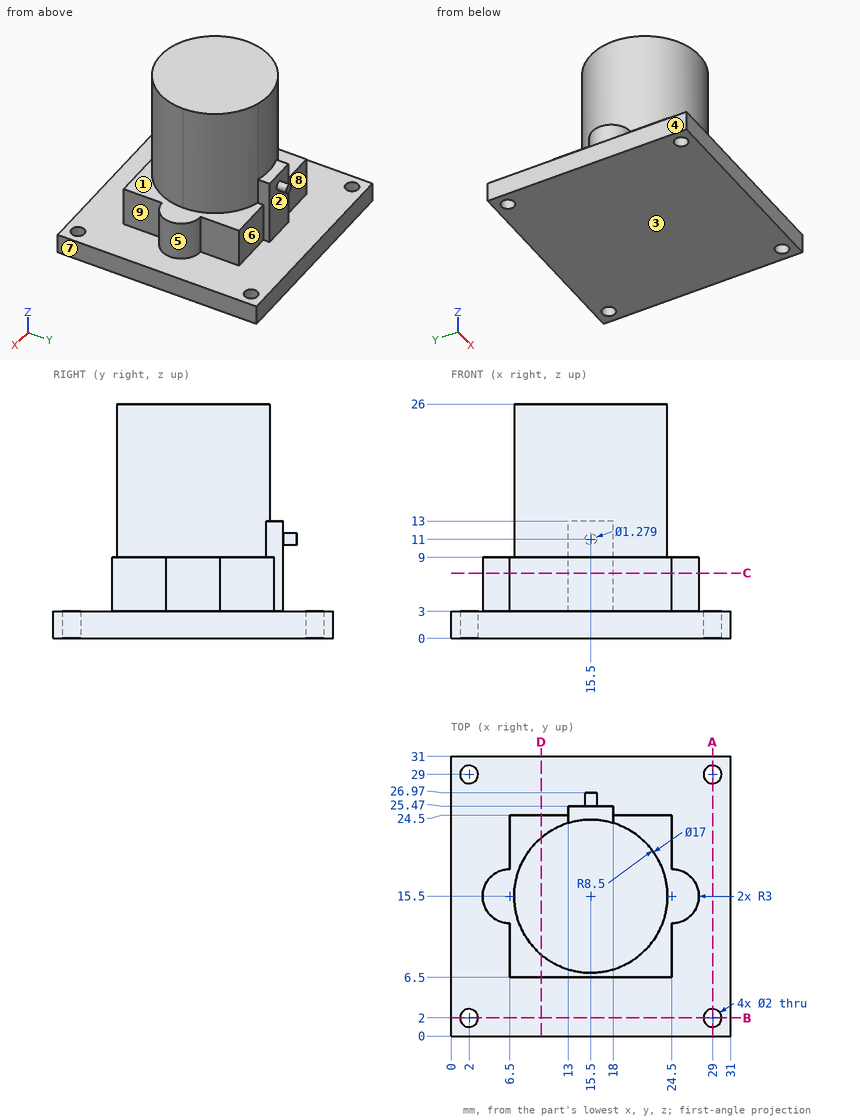
Can you work these out from the drawing? Everything is in mm from the part's minimum corner. A direction names the side the tool comes from. Coordinates: 2 decimals unless noted, no trailing zeros. Loops run counter-clockwise (first coordinate to the right, second up) from the corner with the lowest first, then second, coordinate; pieces in that order, holes last. Notation, with made-up numbers: M 20,22 L 75,22 A22 ccw 75,55 Z; hole C 31.5,5 d6. An arc over 180 degrees is marked long. Put each result on its own line as item: value. Start each with the question number.
(1) Thinking about a two-plate mould opening in Z: for the marked faces 1, 2, 3 and 4, which applies, pulls with the +Z half, pulls with the -Z half, needs draft (parallel to the pull), parting line crosses it, or undercut?
(2) Suppose I cut it at D-D on x = 10. Please give me the cut outline in (y, z).
(3) I need wall thicknesses on line 1 (Y direction, x = 29, z = 0.9); line 2 (X direction, y = 23, z = 7); line 3 (Z direction, x = 21, y = 26). Which ranges of each line are inside material? Lowest first, please. Write a range as from..to.
(4) Suppose I cut it at C-C on z = 7.25. Please give me the cut outline in (x, y), then the cut area to 3 significant figures.
(5) Suppose I cut it at A-A on x = 29. Please give me the cut outline in (y, z).
(6) Will these pins go through, and if not, where does the flat tip stop? P1, Ø8, axis at x = 26, y = 21, coming from the -Z side; P2, Ø3, axis at x = 9.5, z = 7, coming from the +Y side; P3, Ø5.5, axis at x = 16, z = 7, coming from the +Y side; P4, Ø2, axis at y = 24.5, z = 9, coming from the -X side.
(7) For the marked faces 5, 6, 7, 8 and 9, which set-ups out of +Z, -Z, +X, -X, +Y, -Y let a thin tool reach every point of the face, with its end or its side?
Solutions:
1. face 1: pulls with the +Z half
1. face 2: undercut
1. face 3: pulls with the -Z half
1. face 4: needs draft
2. outline: M 0,0 L 31,0 L 31,3 L 24.5,3 L 24.5,9 L 21.98,9 L 21.98,26 L 9.02,26 L 9.02,9 L 6.5,9 L 6.5,3 L 0,3 Z
3. line 1: y = 0..1, 3..28, 30..31
3. line 2: x = 6.5..24.5
3. line 3: z = 0..3
4. outline: M 6.5,6.5 L 24.5,6.5 L 24.5,12.5 A3 ccw 24.5,18.5 L 24.5,24.5 L 18,24.5 L 18,25.47 L 13,25.47 L 13,24.5 L 6.5,24.5 L 6.5,18.5 A3 ccw 6.5,12.5 Z
4. area: 357 mm2
5. outline: M 0,0 L 1,0 L 1,3 L 0,3 Z; M 3,0 L 28,0 L 28,3 L 3,3 Z; M 30,0 L 31,0 L 31,3 L 30,3 Z
6. P1: stops at z = 0
6. P2: stops at y = 24.5
6. P3: stops at y = 25.47
6. P4: stops at x = 6.5
7. face 5: +Z, +X
7. face 6: +Z, +X, +Y
7. face 7: +Z, -Z, +X, +Y, -Y
7. face 8: +Z, -X, +Y
7. face 9: +Z, +X, -Y
